```python
from build123d import *

# Parameters (mm, degrees)
SKETCH_1_R          = 13.05
SKETCH_1_R_2        = 9.5
EXTRUDE_1_DEPTH     = 4
FILLET_1_R          = 3
CUT_EXTRUDE_START   = -10
CUT_EXTRUDE_1_DEPTH = 10
SKETCH_3_R          = 2
CUT_EXTRUDE_2_DEPTH = 10
FILLET_2_R          = 3
SKETCH_4_R          = 2
CUT_EXTRUDE_3_DEPTH = 28
SKETCH_6_R          = 20.45
EXTRUDE_2_DEPTH     = 4
SKETCH_7_R          = 21
EXTRUDE_3_DEPTH     = 4
SKETCH_8_R          = 13.05
CUT_EXTRUDE_4_DEPTH = 4
SKETCH_9_R          = 2
CUT_EXTRUDE_5_DEPTH = 4
FILLET_3_R          = 10


with BuildPart() as part:
    # 草图1 → 凸台-拉伸1 (new body)
    with BuildSketch(Plane.XY):
        with BuildLine():
            Line((-16, 73), (-16, 0))
            ThreePointArc((-16, 0), (-8.327115073, -13.662326103), (7.33239432, -14.220970204))
            Line((7.33239432, -14.220970204), (33.623767545, -0.665023393))
            ThreePointArc((33.623767545, -0.665023393), (41.931803011, 7.070661466), (45, 18))
            Line((45, 18), (45, 73))
            Line((45, 73), (-16, 73))
        make_face()
        with Locations((24, 18)):
            Circle(SKETCH_1_R, mode=Mode.SUBTRACT)
        Circle(SKETCH_1_R_2, mode=Mode.SUBTRACT)
    extrude(amount=EXTRUDE_1_DEPTH)

    # 圆角1
    fillet_1_edges = [part.edges().sort_by_distance(p)[0] for p in [
        (45, 73, 2),
        (-16, 73, 2),
    ]]
    fillet(fillet_1_edges, radius=FILLET_1_R)

    # 草图2 → 切除-拉伸1 (cut)
    with BuildSketch(Plane.XY.offset(4).offset(CUT_EXTRUDE_START)):
        with BuildLine():
            Line((-14.084507501, 7.591221802), (5, 43))
            Line((5, 43), (5, 73))
            Line((5, 73), (-16, 73))
            Line((-16, 73), (-16, 0))
            ThreePointArc((-16, 0), (-15.513737783, 3.914580436), (-14.084507501, 7.591221802))
        make_face()
    extrude(amount=CUT_EXTRUDE_1_DEPTH, mode=Mode.SUBTRACT)

    # 草图3 → 切除-拉伸2 (cut)
    with BuildSketch(Plane.XY.offset(4)):
        with Locations((8.941696856, 26.916137415)):
            Circle(SKETCH_3_R)
        with Locations((19.656832962, 34.952489495)):
            Circle(SKETCH_3_R)
        with Locations((32.916137415, 33.058303144)):
            Circle(SKETCH_3_R)
        with Locations((40.952489495, 22.343167038)):
            Circle(SKETCH_3_R)
        with Locations((39.058303144, 9.083862585)):
            Circle(SKETCH_3_R)
        with Locations((28.343167038, 1.047510505)):
            Circle(SKETCH_3_R)
        with Locations((15.083862585, 2.941696856)):
            Circle(SKETCH_3_R)
        with Locations((7.047510505, 13.656832962)):
            Circle(SKETCH_3_R)
    extrude(amount=-CUT_EXTRUDE_2_DEPTH, mode=Mode.SUBTRACT)

    # 圆角2
    fillet_2_edges = [part.edges().sort_by_distance(p)[0] for p in [
        (5, 43, 2),
        (5, 73, 2),
    ]]
    fillet(fillet_2_edges, radius=FILLET_2_R)

    # 草图4 → 切除-拉伸3 (cut)
    with BuildSketch(Plane.XY.offset(4)):
        with Locations((40, 67.5)):
            Circle(SKETCH_4_R)
        with Locations((10, 67.5)):
            Circle(SKETCH_4_R)
        with Locations((10, 48.5)):
            Circle(SKETCH_4_R)
        with Locations((40, 48.5)):
            Circle(SKETCH_4_R)
    extrude(amount=-CUT_EXTRUDE_3_DEPTH, mode=Mode.SUBTRACT)

    # 草图6 → 凸台-拉伸2 (add)
    with BuildSketch(Plane.XY.offset(4)):
        with Locations((24, 18)):
            Circle(SKETCH_6_R)
    extrude(amount=-EXTRUDE_2_DEPTH)

    # 草图7 → 凸台-拉伸3 (add)
    with BuildSketch(Plane.XY.offset(4)):
        with Locations((25.48, 18)):
            Circle(SKETCH_7_R)
    extrude(amount=-EXTRUDE_3_DEPTH)

    # 草图8 → 切除-拉伸4 (cut)
    with BuildSketch(Plane.XY.offset(4)):
        with Locations((25.48, 18)):
            Circle(SKETCH_8_R)
    extrude(amount=-CUT_EXTRUDE_4_DEPTH, mode=Mode.SUBTRACT)

    # 草图9 → 切除-拉伸5 (cut)
    with BuildSketch(Plane.XY.offset(4)):
        with Locations((10.681592776, 27.341153229)):
            Circle(SKETCH_9_R)
        with Locations((21.621138693, 35.069246891)):
            Circle(SKETCH_9_R)
        with Locations((34.821153229, 32.798407224)):
            Circle(SKETCH_9_R)
        with Locations((42.549246891, 21.858861307)):
            Circle(SKETCH_9_R)
        with Locations((40.278407224, 8.658846771)):
            Circle(SKETCH_9_R)
        with Locations((29.338861307, 0.930753109)):
            Circle(SKETCH_9_R)
        with Locations((16.138846771, 3.201592776)):
            Circle(SKETCH_9_R)
        with Locations((8.410753109, 14.141138693)):
            Circle(SKETCH_9_R)
    extrude(amount=-CUT_EXTRUDE_5_DEPTH, mode=Mode.SUBTRACT)

    # 圆角3
    fillet_3_edges = [part.edges().sort_by_distance(p)[0] for p in [
        (45, 25.744004132, 2),
        (30.087589458, -2.488292252, 2),
    ]]
    fillet(fillet_3_edges, radius=FILLET_3_R)


solid = part.part
```
Can you work these out from the model? Positions are in its coordinate system, mm. A direction names the side the tool comes from. Round coordinates to 2 decimals unless told otherwise and drop trailing zeros. Loops run counter-clockwise (first coordinate to the right, second up) from the corner with the lowest first, then second, coordinate; pieces in that order, holes last. Notation, with made-up numbers: M 3,27 L 61,27 A25 cw 61,56 Z; hole C -23,38 d3. An arc over 180 degrees is marked long. Answer as a JSON object with one key per item and string values. Group by question number.
Q1. Will these pins go through, and if not, where does the flat tip stop? pin 1 (15 mm diameter, centred on x = 0, y = 0, fed in from -Z); pin 2 (2 mm diameter, centred on y = 6.5, z = 3, fed in from -X) (3 decimals); pin 3 (1.5 mm diameter, centred on x = -3.5, z = 2.5, fed in from +Y); pin 4 (5 mm diameter, centred on x = 16.14, y = 3.2, fed in from -Z).
Q2. On a 3-axis mill with a long thin cutter (end or side, diameter ignored), from which of +Z, -Z, +X, -X, +Y, -Y can I reach the whole of each face in a straight line? I mean faces 1 (the flat face through (5, 57, 2)), 2 (the flat face through (45, 48, 2)), 3 (the flat face through (22, 39, 4)). Say none if no direction works.
Q3. Imagine slicing it at B-B, the plane z = 1.85. Count the separate pieces of the cut face and the enclosed holes in it, then the cut area to 3 significant figures.
Q4. We'd pull the mould along X, two halves only. Please class faces 4 (the cylindrical face through (43.825, 7.779, 2.028)), 5 (the cylindrical face through (18.046, 3.802, 2.028)), 6 (the flat face through (22, 39, 0)), 7 (the cylindrical face through (40.923, 46.726, 2.028)): +X half, -X half, draft (parallel to the pull), parting line (faces both ways), or undercut.
Q5. Imagine slicing it at C-C, the plane y = 18. Please give me the cut outline in (x, z).
Q6. Please list where these lines run through material, in increasing order: L1, parallel to Y at x = 28.5, z = 3.1; L2, parallel to Y at x = 10, z = 3.5; L3, parallel to X at y = 26, z = 0.65.
Q7. Imagine slicing it at A-A, the plane x = 0. Please give me the cut outline in (y, z).
Findings:
{
 "1": {"pin 1": "passes through", "pin 2": "stops at x = -15.025", "pin 3": "stops at y = 28.62", "pin 4": "stops at z = 0"},
 "2": {"face 1": "+Z, -Z, -X, +Y", "face 2": "+Z, -Z, +X, +Y", "face 3": "+Z, +X, -X, +Y, -Y"},
 "3": {"separate pieces": "1", "enclosed holes": "14", "area": "2,930 mm2"},
 "4": {"face 4": "+X half", "face 5": "undercut", "face 6": "draft", "face 7": "undercut"},
 "5": {"outline": "M -8.47,0 L 12.43,0 L 12.43,4 L -8.47,4 Z; M 38.53,0 L 46.48,0 L 46.48,4 L 38.53,4 Z"},
 "6": {"L1": "y = -3.31 to -0.88, 2.75 to 5.3, 30.7 to 73", "L2": "y = -12.85 to 12.93, 15.36 to 25.46, 29.22 to 46.5, 50.5 to 65.5, 69.5 to 73", "L3": "x = -4.16 to 9.2, 12.17 to 15.17, 35.79 to 45.11"},
 "7": {"outline": "M -16,0 L -9.5,0 L -9.5,4 L -16,4 Z; M 9.5,0 L 33.72,0 L 33.72,4 L 9.5,4 Z"}
}
